Source: CAD feature listing. Evaluate the final solid. Frame: model axes, mm. A direction names the side the tool comes from. Coordinates: 2 decimals unless noted, no trailing zeros. Write each loop counter-clockwise with the first axis right and the second up, starting at its lowest first coordinate (ties: lowest second). Pieces come first, ordered by that corner, then holes. Notation, with made-up numbers: (58, 32) -> (98, 32) arc R25 cw to (98, 54) -> close; hole circle Ø4 at (73.25, -13.5). An arc over 180 degrees is marked (long way). One line per item, written item: value. Start each with the question number.
1. Mould query, pull axis Z, two halves, no side actions, for faces 5 (the flat face through (0, 32, -15)), 6 (the cylindrical face through (33.96, 16.42, -16.9)), 7 (the flat face through (-13, -25, -30)). Classes: released by +Z, released by -Z, zero draft, split by the parting line, or undercut.
2. Access query for faces 1 (the flat face through (33, 22, -15)), 2 (the flat face through (-38, 11, -11)), 3 (the flat face through (-1, -48, -15)), 4 (the flat face through (-32, 26, -15)). Directions: +Z, -Z, +X, -X, +Y, -Y. A direction counts if a zero-diameter tool reaches every point of the face in a straight line with its end or side. Return the directions, or none.
3. Section query D-D, the plane z = -8.25. Output: boundary loops of the cut face in (x, y), and give its area (3 significant figures).
4. Section query A-A, the plane y = 0. Output: boundary loops of the cut face in (x, z).
5. Section query C-C, the plane x = 0. Output: boundary loops of the cut face in (y, z), and give its area (3 significant figures).
6. First-contact query: P1, Ø2.5, axis at y = 24.5, z = -19.5, coming from the -X side; P2, Ø14, axis at x = -43.5, z = -14.5, coming from the +Y side; P3, Ø15.5, axis at x = -40, z = -12, coming from the +Y side. Flat tips, straight axial feed; report the tip coordinate or a pass-through.
7. Section query B-B, the plane z = -15. State how many separate pieces and enclosed holes the cut face has, and give its area (3 significant figures).
8. Line query: line 1 (X direction, y = -34, z = -15); line 2 (Z direction, x = 43, y = -9.5); line 3 (X direction, y = 18.5, z = -15). Output: solid intervals per line, ascending.
from build123d import *

# Parameters (mm, degrees)
BOSS_EXTRUDE1_DEPTH = 30
SKETCH4_R           = 26
CUT_EXTRUDE1_DEPTH  = 30


with BuildPart() as part:
    # Sketch1 → Boss-Extrude1 (new body)
    with BuildSketch(Plane.XY):
        Polygon((-53, -46.08), (-51.08, -48), (51.08, -48), (53, -46.08), (53, 20.08), (51.08, 22), (32, 22), (32, 30), (30, 32), (-30, 32), (-32, 30), (-32, 22), (-51.08, 22), (-53, 20.08), align=None)
    extrude(amount=-BOSS_EXTRUDE1_DEPTH)

    # Sketch2 → Cut-Revolve1 (revolve, cut)
    with BuildSketch(Plane(origin=(42.5, 0, 0), x_dir=(0, 0, -1), z_dir=(1, 0, 0)), mode=Mode.PRIVATE) as cut_revolve1_sk:
        Polygon((15, 22), (23.75, 22), (23.75, 11), (20.5, 11), (20.5, -48), (15, -48), align=None)
    revolve(cut_revolve1_sk.sketch.rotate(Axis((42.5, -48, -15), (0, 1, 0)), 180), axis=Axis((42.5, -48, -15), (0, 1, 0)), mode=Mode.SUBTRACT)

    # Sketch3 → Cut-Revolve2 (revolve, cut)
    with BuildSketch(Plane(origin=(-42.5, 0, 0), x_dir=(0, 0, -1), z_dir=(1, 0, 0)), mode=Mode.PRIVATE) as cut_revolve2_sk:
        Polygon((15, 22), (23.75, 22), (23.75, 11), (20.5, 11), (20.5, -48), (15, -48), align=None)
    revolve(cut_revolve2_sk.sketch.rotate(Axis((-42.5, -48, -15), (0, 1, 0)), 180), axis=Axis((-42.5, -48, -15), (0, 1, 0)), mode=Mode.SUBTRACT)

    # Sketch4 → Cut-Extrude1 (cut)
    with BuildSketch(Plane.XY):
        Circle(SKETCH4_R)
    extrude(amount=-CUT_EXTRUDE1_DEPTH, mode=Mode.SUBTRACT)


solid = part.part
Computed values:
1. face 5: zero draft
1. face 6: undercut
1. face 7: released by -Z
2. face 1: +Z, -Z, +X, +Y
2. face 2: +Y
2. face 3: +Z, -Z, +X, -X, -Y
2. face 4: +Z, -Z, -X, +Y
3. outline: (-53, -46.08) -> (-51.08, -48) -> (51.08, -48) -> (53, -46.08) -> (53, 20.08) -> (51.08, 22) -> (48.07, 22) -> (48.07, 11) -> (36.93, 11) -> (36.93, 22) -> (32, 22) -> (32, 30) -> (30, 32) -> (-30, 32) -> (-32, 30) -> (-32, 22) -> (-36.93, 22) -> (-36.93, 11) -> (-48.07, 11) -> (-48.07, 22) -> (-51.08, 22) -> (-53, 20.08) -> close; hole circle Ø52 at (0, 0)
3. area: 5,680 mm²
4. outline: (-53, -30) -> (-26, -30) -> (-26, 0) -> (-53, 0) -> close; (26, -30) -> (53, -30) -> (53, 0) -> (26, 0) -> close; hole circle Ø11 at (-42.5, -15); hole circle Ø11 at (42.5, -15)
5. outline: (-48, -30) -> (-26, -30) -> (-26, 0) -> (-48, 0) -> close; (26, -30) -> (32, -30) -> (32, 0) -> (26, 0) -> close
5. area: 840 mm²
6. P1: stops at x = -32
6. P2: stops at y = 11
6. P3: stops at y = 22
7. separate pieces: 3
7. enclosed holes: 1
7. area: 4,240 mm²
8. line 1: x = -53 to -48, -37 to 37, 48 to 53
8. line 2: z = -30 to -20.48, -9.52 to 0
8. line 3: x = -53 to -51.25, -33.75 to -18.27, 18.27 to 33.75, 51.25 to 53
